Autodesk Inventor part; units mm, degrees
ref_plane "YZ Plane" through (0, 0, 0) normal (1, 0, 0) x (0, 1, 0)
ref_plane "XZ Plane" through (0, 0, 0) normal (0, 1, 0) x (-1, 0, 0)
ref_plane "XY Plane" through (0, 0, 0) normal (0, 0, 1) x (1, 0, 0)
sketch "Sketch1" plane through (0, 0, 0) normal (0, 0, 1) x (1, 0, 0)
  line L0 (0, 0) -> (0, 50.5)
  line L1 (0, 50.5) -> (2.85, 50.5)
  line L2 (2.85, 50.5) -> (2.85, 47.9)
  line L3 (2.85, 47.9) -> (4, 47.9)
  line L4 (4, 47.9) -> (4, 6)
  line L5 (4, 6) -> (1.5, 6)
  line L6 (1.5, 6) -> (1.5, 0)
  line L7 (1.5, 0) -> (0, 0)
  dimension "d0" = 3
  dimension "d1" = 6
  dimension "d2" = 50.5
  dimension "d3" = 5.7
  dimension "d4" = 8
  dimension "d5" = 2.6
revolve "Revolution1" add sketch "Sketch1" angle 360 about axis through (0, 0, 0) along (0, 1, 0)
properties part number "Pok X-Carriage Top Support" material "ABS Plastic"
Source: CAD feature listing. Evaluate the final solid. Frame: model axes, mm. A direction names the side the tool comes from. Give positions to 0.01 mm unless a question says otherwise; leave off trailing zeros. Write each loop counter-clockwise with the first axis right and the second up, starting at its lowest first coordinate (ties: lowest second). Pieces come first, ordered by that corner, then holes. Notation, with made-up numbers: (30, 33.5) -> (58, 33.5) arc R15 cw to (58, 39.5) -> close; hole circle Ø2 at (56.25, 89). An arc over 180 degrees is marked (long way). Return JSON: item names as keys, results as strings. Group by question number.
1. Material intervals for line 1 (Y direction, x = 2.25, z = 0.25); line 2 (Z direction, x = -0.25, y = 47); line 3 (Y direction, x = 2.5, z = 1.5), sorted ascending. Write a range as from..to.
2. Section B-B, the plane x = 0. Output: boundary loops of the cut face in (y, z).
3. Access query for faces 1 (the face through (2, 6, 0)), 2 (the face through (0, 0, 0)), 3 (the face through (-2.262, 49.182, -1.734)). Directions: +Z, -Z, +X, -X, +Y, -Y. A direction counts if a zero-diameter tool reaches every point of the face in a straight line with its end or side. Return the directions, or none.
4. Section D-D, the plane x = -2. Output: boundary loops of the cut face in (y, z), then the cut area to 3 significant figures.
5. Section C-C, the plane y = 4.5. Output: boundary loops of the cut face in (x, z).
6. Section A-A, the plane z = 0. Output: boundary loops of the cut face in (x, y), then the cut area to 3 significant figures.
7. Pin query (flat end, axial travel): pin 1 Ø4 at (y, z) = (26, 2.5) entering from -X; pin 2 Ø4 at (x, z) = (0, 0.5) entering from -Y; pin 3 Ø1.5 at (x, z) = (2.5, 3) entering from +Y; pin 4 Ø2 at (x, z) = (2, 3) entering from -Y. Return the tip coordinate at first contact, or that it passes through.
Determined:
{
 "1": {"line 1": "y = 6..50.5", "line 2": "z = -3.99..3.99", "line 3": "y = 6..47.9"},
 "2": {"outline": "(0, -1.5) -> (6, -1.5) -> (6, -4) -> (47.9, -4) -> (47.9, -2.85) -> (50.5, -2.85) -> (50.5, 2.85) -> (47.9, 2.85) -> (47.9, 4) -> (6, 4) -> (6, 1.5) -> (0, 1.5) -> close"},
 "3": {"face 1": "-Y", "face 2": "+Z, -Z, +X, -X, -Y", "face 3": "+Y"},
 "4": {"outline": "(6, -3.46) -> (47.9, -3.46) -> (47.9, -2.03) -> (50.5, -2.03) -> (50.5, 2.03) -> (47.9, 2.03) -> (47.9, 3.46) -> (6, 3.46) -> close", "area": "301 mm2"},
 "5": {"outline": "circle Ø3 at (0, 0)"},
 "6": {"outline": "(-4, 6) -> (-1.5, 6) -> (-1.5, 0) -> (1.5, 0) -> (1.5, 6) -> (4, 6) -> (4, 47.9) -> (2.85, 47.9) -> (2.85, 50.5) -> (-2.85, 50.5) -> (-2.85, 47.9) -> (-4, 47.9) -> close", "area": "368 mm2"},
 "7": {"pin 1": "stops at x = -3.97", "pin 2": "stops at y = 0", "pin 3": "stops at y = 47.9", "pin 4": "stops at y = 6"}
}
